Could you check a few things on this model? Use its own coordinates, in mm. A direction names the side the tool comes from. Give positions to 0.01 mm unless a question says otherwise; leave off trailing zeros. Loops run counter-clockwise (first coordinate to the right, second up) from the corner with the lowest first, then second, coordinate; pieces in that order, holes last. Notation, with made-up numbers: M -8,55 L 0,55 A23 cw 0,67 Z; hole C -24,57.5 d4. An arc over 180 degrees is marked long. Return JSON: item names as keys, results as strings. Group by question number.
1. If we mould it in two halves opening along Y, with no side actions, what happens to faces 1 (the cylindrical face through (3.19, -12.63, -45.51)), 2 (the cylindrical face through (5.43, 22.68, 47.94)), 3 (the flat face through (5, -25.4, -1)), 4 (the flat face through (6.3, -12, 41))? For each: +Y half, -Y half, draft (parallel to the pull), parting line (faces both ways), or undercut.
2. For faces 5 (the flat face through (6.3, -12, -41)), 6 (the cylindrical face through (7.8, 15.7, 37.9)), which set-ups out of +Z, -Z, +X, -X, +Y, -Y let a thin tool reach every point of the face, with its end or its side?
3. If we section it at C-C (z = 15.5): State how many separate pieces and enclosed holes the cut face has, plus the area to 3 significant figures.
4. For pin 1 (5.5 mm diameter, centred on y = -16.5, z = -43.5, fed in from -X); pin 2 (6 mm diameter, centred on y = -15.49, z = -15.49, fed in from -X), each with a flat end and sliding along its axis, tell me the tip position at first contact or that it passes through.
5. If we section it at B-B (z = -8): Write out the boundary of the cut face in (x, y) (1 decimal), plus the area to 3 significant figures.
6. If we section it at A-A (y = 0): Write out the boundary of the cut face in (x, z) (1 decimal).
7. Please list where these lines run through material, in increasing order: line 1 (Z direction, x = 4, y = -15.5); line 2 (Y direction, x = 8, z = -42); line 3 (Y direction, x = 4.5, z = -8).
Autodesk Inventor part; units mm, degrees
ref_plane "YZ Plane" through (0, 0, 0) normal (1, 0, 0) x (0, 1, 0)
ref_plane "XZ Plane" through (0, 0, 0) normal (0, 1, 0) x (-1, 0, 0)
ref_plane "XY Plane" through (0, 0, 0) normal (0, 0, 1) x (1, 0, 0)
sketch "Sketch1" plane through (0, 0, 0) normal (1, 0, 0) x (0, 1, 0)
  line L0 (-25.4, 50.8) -> (25.4, 50.8)
  line L1 (25.4, 50.8) -> (25.4, -50.8)
  line L2 (25.4, -50.8) -> (-25.4, -50.8)
  line L3 (-25.4, -50.8) -> (-25.4, 50.8)
  line L4 (-25.4, 50.8) -> (25.4, -50.8) construction
  line L5 (25.4, 50.8) -> (-25.4, -50.8) construction
  point P0 (0, 0)
  dimension "d0" = 50.8
  dimension "d1" = 101.6
extrude "Extrusion1" add sketch "Sketch1" along normal blind 9.175
fillet "Fillet1" radius 9.525 4 edges at (4.5875, 25.4, 50.8) (4.5875, -25.4, 50.8) (4.5875, -25.4, -50.8) (4.5875, 25.4, -50.8)
sketch "Sketch2" plane through (0, 0, 0) normal (-1, 0, 0) x (0, 0, 1)
  circle A0 centre (-8, 0) radius 8
  point P0 (0, 0)
  dimension "d5" = 16
extrude "Extrusion2" cut sketch "Sketch2" against normal through all
sketch "Sketch3" plane through (0, 0, 0) normal (-1, 0, 0) x (0, 0, 1)
  circle A0 centre (-8, 0) radius 8
  arc A1 (-41.275, 25.4) -> (-50.8, 15.875) centre (-41.275, 15.875) ccw
  line L0 (-50.8, -15.875) -> (-50.8, 15.875)
  arc A2 (-50.8, -15.875) -> (-41.275, -25.4) centre (-41.275, -15.875) ccw
  line L1 (41.275, -25.4) -> (-41.275, -25.4)
  arc A3 (41.275, -25.4) -> (50.8, -15.875) centre (41.275, -15.875) ccw
  line L2 (50.8, 15.875) -> (50.8, -15.875)
  arc A4 (50.8, 15.875) -> (41.275, 25.4) centre (41.275, 15.875) ccw
  line L3 (-41.275, 25.4) -> (41.275, 25.4)
  point P0 (0, 0)
hole "Hole1" at (0, 15.875, -41.275) at (0, -15.875, -41.275) at (0, -15.875, 41.275) at (0, 15.875, 41.275) direction (1, 0, 0) diameter 6.7564 end through all counterbore diameter 10.668 counterbore depth 6.3
chamfer "Chamfer1" distance 1.5875 angle 45 8 edges at (0, 0, -50.8) (0, 22.6102, -48.0102) (0, 25.4, 0) (0, 22.6102, 48.0102) (0, 0, 50.8) (0, -22.6102, 48.0102) (0, -25.4, 0) (0, -22.6102, -48.0102)
sketch "Sketch4" plane through (0, 0, 0) normal (-1, 0, 0) x (0, 0, 1)
  circle A0 centre (15.4856, 15.4856) radius 1.621
  circle A1 centre (-15.4856, 15.4856) radius 1.621
  circle A2 centre (-15.4856, -15.4856) radius 1.621
  circle A3 centre (15.4856, -15.4856) radius 1.621
  point P0 (0, 0)
hole "Hole2" at (0, 15.4856, -15.4856) at (0, 15.4856, 15.4856) at (0, -15.4856, 15.4856) at (0, -15.4856, -15.4856) direction (1, 0, 0) diameter 4.6 end through all countersink diameter 8.6 countersink angle 90
properties part number "NASA-20-MM-MP-01" material "Aluminum 6061"
Answer:
{
 "1": {"face 1": "undercut", "face 2": "+Y half", "face 3": "-Y half", "face 4": "undercut"},
 "2": {"face 5": "-X", "face 6": "+X, -X"},
 "3": {"separate pieces": "3", "enclosed holes": "0", "area": "371 mm²"},
 "4": {"pin 1": "stops at x = 6.3", "pin 2": "stops at x = 1.29"},
 "5": {"outline": "M 0,-23.8 L 1.6,-25.4 L 9.2,-25.4 L 9.2,-8 L 0,-8 Z; M 0,8 L 9.2,8 L 9.2,25.4 L 1.6,25.4 L 0,23.8 Z", "area": "317 mm²"},
 "6": {"outline": "M 0,-49.2 L 1.6,-50.8 L 9.2,-50.8 L 9.2,-16 L 0,-16 Z; M 0,0 L 9.2,0 L 9.2,50.8 L 1.6,50.8 L 0,49.2 Z"},
 "7": {"line 1": "z = -50.8 to -46.6, -35.95 to -17.79, -13.19 to 13.19, 17.79 to 35.95, 46.6 to 50.8", "line 2": "y = -25.37 to -19.17, -12.58 to 12.58, 19.17 to 25.37", "line 3": "y = -25.4 to -8, 8 to 25.4"}
}
